Geometry check sheet. Reference: the model listing, model coordinates, mm. A direction names the side the tool comes from. Round coordinates to 2 decimals unless told otherwise and drop trailing zeros. Order: outer loops, then holes, each group sorted by start corner. A loop starts at its lowest first (then second) coordinate and runs counter-clockwise, first axis right, second up. Notation, with made-up numbers: (13, -10) - (28, -10) arc R12 ccw to (28, 10) - close; hole circle Ø7 at (77.25, 85.5). An arc over 180 degrees is marked (long way). Return JSON: item names as keys, results as strings. Group by question number.
Q1. Sectioned sample at B-B, the plane x = 1.25. Record the cut outline in (y, z).
Q2. Sectioned sample at A-A, the plane z = 1.75. Record the cut outline in (x, y), then the cut area to 3 significant figures.
Q3. Sectioned sample at D-D, the plane x = -4. Record the cut outline in (y, z), then the cut area to 3 significant figures.
Q4. Draft check along X on faces 3 (the cylindrical face through (3.958, 0.561, 2.958)), 4 (the cylindrical face through (4.08, 0.4, 3.55)), 5 (the cylindrical face through (-4.1, 0.42, 3.55)). Enter one of: pulls with the +X half, pulls with the -X half, needs draft (parallel to the pull), parting line crosses it, or undercut.
Q5. Material ranges on line 1 along Y through (x, z) = (2.5, 0.75); line 2 along X through (y, z) = (1.7, 3.5); line 3 along X through (y, z) = (2.25, 5), recorded low to high.
Q6. Tool access check on faces 1 (the cylindrical face through (-3.958, 2.439, 2.958)), 2 (the flat face through (0, 2, 7)). Record the directions out of +Z, -Z, +X, -X, +Y, -Y that give a thin tool (end or side, any length) a straight path to the whole face; none if there is none.
Q7. Sectioned sample at C-C, the plane y = 0.35. Record the cut outline in (x, z).
Autodesk Inventor part; units mm, degrees
ref_plane "YZ Plane" through (0, 0, 0) normal (1, 0, 0) x (0, 1, 0)
ref_plane "XZ Plane" through (0, 0, 0) normal (0, 1, 0) x (-1, 0, 0)
ref_plane "XY Plane" through (0, 0, 0) normal (0, 0, 1) x (1, 0, 0)
sketch "Sketch1" plane through (0, 0, 0) normal (0, 0, 1) x (1, 0, 0)
  line L0 (-4.5, 0) -> (4.5, 0)
  line L1 (4.5, 0) -> (4.5, 3)
  line L2 (4.5, 3) -> (-4.5, 3)
  line L3 (-4.5, 3) -> (-4.5, 0)
  line L4 (-4.5, 0) -> (4.5, 3) construction
  line L5 (4.5, 0) -> (-4.5, 3) construction
  point P0 (0, 0)
  point P1 (0, 0)
  dimension "d0" = 9
  dimension "d1" = 3
extrude "Extrusion1" add sketch "Sketch1" along normal blind 7
fillet "Fillet1" radius 1.4 4 edges at (4.5, 3, 3.5) (-4.5, 3, 3.5) (-4.5, 0, 3.5) (4.5, 0, 3.5)
sketch "Sketch2" plane through (0, 0, 0) normal (0, 0, -1) x (-1, 0, 0)
  arc A0 (-4.5, 1.4) -> (-3.1, 0) centre (-3.1, 1.4) ccw
  line L0 (3.1, 0) -> (-3.1, 0)
  arc A1 (3.1, 0) -> (4.5, 1.4) centre (3.1, 1.4) ccw
  line L1 (4.5, 1.6) -> (4.5, 1.4)
  arc A2 (4.5, 1.6) -> (3.1, 3) centre (3.1, 1.6) ccw
  line L2 (-3.1, 3) -> (3.1, 3)
  arc A3 (-3.1, 3) -> (-4.5, 1.6) centre (-3.1, 1.6) ccw
  line L3 (-4.5, 1.4) -> (-4.5, 1.6)
  arc A4 (4.3, 1.6) -> (3.1, 2.8) centre (3.1, 1.6) ccw
  line L4 (4.3, 1.6) -> (4.3, 1.4)
  arc A5 (3.1, 0.2) -> (4.3, 1.4) centre (3.1, 1.4) ccw
  line L5 (3.1, 0.2) -> (-3.1, 0.2)
  arc A6 (-4.3, 1.4) -> (-3.1, 0.2) centre (-3.1, 1.4) ccw
  line L6 (-4.3, 1.4) -> (-4.3, 1.6)
  arc A7 (-3.1, 2.8) -> (-4.3, 1.6) centre (-3.1, 1.6) ccw
  line L7 (-3.1, 2.8) -> (3.1, 2.8)
  line L8 (-3.5, 1.85) -> (3.5, 1.85)
  line L9 (3.5, 1.85) -> (3.5, 1.15)
  line L10 (3.5, 1.15) -> (-3.5, 1.15)
  line L11 (-3.5, 1.15) -> (-3.5, 1.85)
  line L12 (-3.5, 1.85) -> (3.5, 1.15) construction
  line L13 (3.5, 1.85) -> (-3.5, 1.15) construction
  point P0 (0, 0)
  point P1 (0, 1.5)
  point P2 (4.5, 1.5)
  point P3 (0, 0)
  dimension "d5" = 0.2
  dimension "d6" = 7
  dimension "d7" = 0.7
extrude "Extrusion2" cut sketch "Sketch2" against normal blind 6 contours L4 A5 L5 A6 L6 A7 L7 A4
fillet "Fillet2" radius 0.3 4 edges at (3.5, 1.15, 3) (3.5, 1.85, 3) (-3.5, 1.15, 3) (-3.5, 1.85, 3)
properties part number "USB_C"
Reply:
{
 "1": {"outline": "(0, 0) - (0.2, 0) - (0.2, 6) - (1.15, 6) - (1.15, 0) - (1.85, 0) - (1.85, 6) - (2.8, 6) - (2.8, 0) - (3, 0) - (3, 7) - (0, 7) - close"},
 "2": {"outline": "(-4.5, 1.4) arc R1.4 ccw to (-3.1, 0) - (3.1, 0) arc R1.4 ccw to (4.5, 1.4) - (4.5, 1.6) arc R1.4 ccw to (3.1, 3) - (-3.1, 3) arc R1.4 ccw to (-4.5, 1.6) - close; (-3.5, 1.45) arc R0.3 ccw to (-3.2, 1.15) - (3.2, 1.15) arc R0.3 ccw to (3.5, 1.45) - (3.5, 1.55) arc R0.3 ccw to (3.2, 1.85) - (-3.2, 1.85) arc R0.3 ccw to (-3.5, 1.55) - close; hole (-4.3, 1.4) arc R1.2 ccw to (-3.1, 0.2) - (3.1, 0.2) arc R1.2 ccw to (4.3, 1.4) - (4.3, 1.6) arc R1.2 ccw to (3.1, 2.8) - (-3.1, 2.8) arc R1.2 ccw to (-4.3, 1.6) - close", "area": "9.02 mm^2"},
 "3": {"outline": "(0.33, 0) - (0.61, 0) - (0.61, 6) - (2.39, 6) - (2.39, 0) - (2.67, 0) - (2.67, 7) - (0.33, 7) - close", "area": "5.69 mm^2"},
 "4": {"face 3": "undercut", "face 4": "pulls with the +X half", "face 5": "pulls with the -X half"},
 "5": {"line 1": "0 to 0.2, 1.15 to 1.85, 2.8 to 3", "line 2": "-4.5 to -4.3, -3.46 to 3.46, 4.3 to 4.5", "line 3": "-4.34 to -4.11, 4.11 to 4.34"},
 "6": {"face 1": "-Z", "face 2": "+Z, +X, -X, +Y, -Y"},
 "7": {"outline": "(-4.03, 0) - (-3.68, 0) - (-3.68, 6) - (3.68, 6) - (3.68, 0) - (4.03, 0) - (4.03, 7) - (-4.03, 7) - close"}
}
